Autodesk Fusion 360 part; units mm, degrees
sketch "Sketch1" plane through (0, 0, 0) normal (0, 1, 0) x (1, 0, 0)
  circle A0 centre (0, 0) radius 1.5
  circle A1 centre (50.8, -15.2) radius 1.5
  circle A2 centre (50.8, -43.1) radius 1.5
  circle A3 centre (-1.3, -48.2) radius 1.5
  line L0 (-10, 8.8) -> (57, 8.8)
  line L1 (57, 8.8) -> (57, -58.2)
  line L2 (57, -58.2) -> (-10, -58.2)
  line L3 (-10, -58.2) -> (-10, 8.8)
  circle A4 centre (50.8, -15.2) radius 2.5
  circle A5 centre (50.8, -43.1) radius 2.5
  circle A6 centre (-1.3, -48.2) radius 2.5
  circle A7 centre (0, 0) radius 2.5
  dimension "d1" = 3
  dimension "d2" = 3
  dimension "d3" = 50.8
  dimension "d4" = 15.2
  dimension "d5" = 3
  dimension "d6" = 27.9
  dimension "d7" = 3
  dimension "d8" = 5.1
  dimension "d9" = 1.3
  dimension "d10" = 67
  dimension "d11" = 67
  dimension "d12" = 10
  dimension "d13" = 10
  dimension "d16" = 5
  dimension "d17" = 5
  dimension "d18" = 5
  dimension "d19" = 5
extrude "Extrude1" add sketch "Sketch1" along normal blind 13 contours A0 | A1 | A2 | A3 makes body 1 at (51.2777, 8.6667, 13.7781) makes body 2 at (52.0799, 8.6667, 42.3178) makes body 3 at (1.4925, 8.6667, 0.1494) makes body 4 at (-2.6822, 8.6667, 48.7827)
extrude "Extrude3" add sketch "Sketch1" along normal blind 10 contours A5 bodies 2
extrude "Extrude4" add sketch "Sketch1" along normal blind 10 contours A4 bodies 1
extrude "Extrude5" add sketch "Sketch1" along normal blind 10 contours A6 bodies 4
extrude "Extrude6" add sketch "Sketch1" along normal blind 10 contours A7 bodies 3
extrude "Extrude7" add sketch "Sketch1" along normal blind 3 contours L0 L1 L2 L3 bodies 1 2 3 4
sketch "Sketch2" plane through (0, 3, 0) normal (0, 1, 0) x (-1, 0, 0)
  circle A0 centre (0, 0) radius 2.5
  circle A1 centre (-50.8, 15.2) radius 2.5
  circle A2 centre (1.3, 48.2) radius 2.5
  circle A3 centre (-50.8, 43.1) radius 2.5
  line L0 (10, 58.2) -> (-57, 58.2)
  line L1 (-57, 58.2) -> (-57, -8.8)
  line L2 (-57, -8.8) -> (10, -8.8)
  line L3 (10, -8.8) -> (10, 58.2)
  circle A4 centre (-6.7207, 2.6289) radius 3
  circle A5 centre (-18.3874, 2.6289) radius 3
  circle A6 centre (-30.054, 2.6289) radius 3
  circle A7 centre (-41.7207, 2.6289) radius 3
  circle A8 centre (-6.7207, 13.8789) radius 3
  circle A9 centre (-18.3874, 13.8789) radius 3
  circle A10 centre (-30.054, 13.8789) radius 3
  circle A11 centre (-41.7207, 13.8789) radius 3
  circle A12 centre (-6.7207, 25.1289) radius 3
  circle A13 centre (-18.3874, 25.1289) radius 3
  circle A14 centre (-30.054, 25.1289) radius 3
  circle A15 centre (-41.7207, 25.1289) radius 3
  circle A16 centre (-6.7207, 36.3789) radius 3
  circle A17 centre (-18.3874, 36.3789) radius 3
  circle A18 centre (-30.054, 36.3789) radius 3
  circle A19 centre (-41.7207, 36.3789) radius 3
  circle A20 centre (-6.7207, 47.6289) radius 3
  circle A21 centre (-18.3874, 47.6289) radius 3
  circle A22 centre (-30.054, 47.6289) radius 3
  circle A23 centre (-41.7207, 47.6289) radius 3
  dimension "d37" = 6
  dimension "d40" = -35
  dimension "d41" = 45
extrude "Extrude8" cut sketch "Sketch2" against normal blind 3 contours A4 | A5 | A6 | A7 | A8 | A9 | A10 | A11 | A12 | A13 | A14 | A15 | A16 | A17 | A18 | A19 | A20 | A21 | A22 | A23 bodies 1
extrude "Extrude2" [suppressed]
equation "d1 = HoleSize"
equation "d2 = HoleSize"
equation "d5 = HoleSize"
equation "d7 = HoleSize"
equation "HoleSize = 3 mm"
equation "PostSize = 5 mm"
equation "d16 = PostSize"
equation "d17 = PostSize"
equation "d18 = PostSize"
equation "d19 = PostSize"
equation "PostHeight = 10 mm"
equation "PegHeight = 3 mm"
equation "d22 = PostHeight + PegHeight"
equation "d24 = PostHeight"
equation "d26 = PostHeight"
equation "d28 = PostHeight"
equation "d30 = PostHeight"
equation "d32 = PostHeight"
equation "PlatformHeight = 3 mm"
equation "d35 = PlatformHeight"
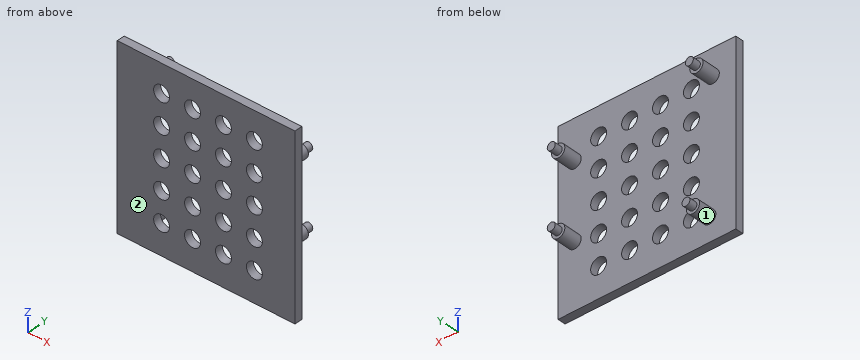
Geometry: final body of the model. Coordinates: model frame, mm. Face numbers are marked on the shaded views. Round coordinates to 2 decimals unless told otherwise and drop trailing zeros. Loops run counter-clockwise (first coordinate to the right, second up) from the corner with the lowest first, then second, coordinate; pieces in that order, holes last. Notation, with made-up numbers: (52, 13) -> (73, 13) arc R4 cw to (73, 20) -> close; hole circle Ø4 at (9.25, 6). An arc over 180 degrees is marked (long way). Write each question's results on one line, items separated by ' | '.
Item 1: Line query: probe 1 along Z at (x, y) = (4, 1.75); probe 2 along Y at (x, z) = (16, 40.5); probe 3 along Y at (x, z) = (50.5, 13). Output: solid intervals per line, ascending. Write a range as [from, to].
Answers below:
probe 1: z = [-8.8, 1.36], [3.89, 12.61], [15.14, 23.86], [26.39, 35.11], [37.64, 46.36], [48.89, 58.2] | probe 2: y = [0, 3] | probe 3: y = [0, 10]
Item 2: Cut plane C-C on y = 7.75. Return the cut outline in (x, z).
Answers below:
outline: circle Ø5 at (-1.3, 48.2); circle Ø5 at (0, 0); circle Ø5 at (50.8, 15.2); circle Ø5 at (50.8, 43.1)
Item 3: Cut plane A-A on z = 38.5. Return the cut outline in (x, y), and give its area (3 significant figures).
Answers below:
outline: (-10, 0) -> (4.6, 0) -> (4.6, 3) -> (-10, 3) -> close; (8.84, 0) -> (16.27, 0) -> (16.27, 3) -> (8.84, 3) -> close; (20.51, 0) -> (27.93, 0) -> (27.93, 3) -> (20.51, 3) -> close; (32.18, 0) -> (39.6, 0) -> (39.6, 3) -> (32.18, 3) -> close; (43.84, 0) -> (57, 0) -> (57, 3) -> (43.84, 3) -> close | area: 150 mm²
Item 4: Pull-direction query (Z, two-part tool) for the marked faces 1 and 2; classes: pulls with the +Z half, pulls with the -Z half, needs draft (parallel to the pull), parting line crosses it, or undercut.
Answers below:
face 1: undercut | face 2: needs draft
Item 5: Cut plane B-B on y = 1.75. State how many separate pieces and enclosed holes the cut face has, and give its area (3 significant figures).
Answers below:
separate pieces: 1 | enclosed holes: 20 | area: 3,920 mm²
Item 6: Cut plane D-D on z = 19. Return the cut outline in (x, y), and give its area (3 significant figures).
Answers below:
outline: (-10, 0) -> (57, 0) -> (57, 3) -> (-10, 3) -> close | area: 201 mm²
Item 7: Pin query (flat end, axial travel): pin 1 Ø1 at (x, z) = (18.5, 47) entering from +Y; pin 2 Ø7 at (x, z) = (41.72, 47.63) entering from +Y. Return the tip coordinate at first contact, or that it passes through.
Answers below:
pin 1: passes through | pin 2: stops at y = 3
